Autodesk Inventor part; units mm, degrees
ref_plane "YZ Plane" through (0, 0, 0) normal (1, 0, 0) x (0, 1, 0)
ref_plane "XZ Plane" through (0, 0, 0) normal (0, 1, 0) x (-1, 0, 0)
ref_plane "XY Plane" through (0, 0, 0) normal (0, 0, 1) x (1, 0, 0)
sketch "Esboço2" plane through (0, 0, 0) normal (0, 0, 1) x (1, 0, 0)
  line L0 (0, 0) -> (57, 0)
  line L1 (57, 0) -> (57, 125)
  line L2 (74, 135) -> (74, 161)
  line L3 (74, 161) -> (73, 161)
  line L4 (57, 125) -> (74, 135)
  line L5 (73, 135.5719) -> (56, 125.5719)
  line L6 (56, 125.5719) -> (56, 1)
  line L7 (56, 1) -> (1, 1)
  line L8 (1, 1) -> (0, 1)
  line L9 (0, 1) -> (0, 0)
  line L10 (0, 45.3298) -> (0, 108.1085)
  line L11 (73, 160) -> (73, 161)
  line L12 (73, 138.8946) -> (0.9659, 119.5931)
  line L13 (73, 138.8946) -> (148.5752, 138.8946) construction
  line L14 (0.9659, 118.5931) -> (73, 137.8946)
  line L15 (73, 160) -> (73, 138.8946)
  line L16 (73, 137.8946) -> (73, 135.5719)
  line L17 (0.9659, 119.5931) -> (0.9659, 118.5931)
  dimension "d0" = 57
  dimension "d1" = 125
  dimension "d5" = 26
  dimension "d8" = 1
  dimension "d9" = 165
revolve "Revolução1" add sketch "Esboço2" angle 360 about axis through (0, 45.3298, 0) along (0, 1, 0)
sketch "Esboço3" plane through (0, 0, 0) normal (0, -1, 0) x (1, 0, 0)
  circle A0 centre (0, 0) radius 2.5
  dimension "d13" = 5
extrude "Extrusão1" cut sketch "Esboço3" against normal blind 10
sketch "Esboço4" plane through (0, 0, 0) normal (0, -1, 0) x (1, 0, 0)
  circle A0 centre (0, 0) radius 57
  line L0 (107, 0) -> (107, 32.5)
  line L1 (107, 32.5) -> (107, -32.5)
  line L2 (107, -32.5) -> (27, -32.5)
  line L3 (27, -32.5) -> (107, -32.5)
  line L4 (107, -32.5) -> (107, 32.5)
  line L5 (107, 32.5) -> (27, 32.5)
  line L6 (27, 32.5) -> (27, -32.5)
  point P0 (0, 0)
  dimension "d17" = 32.5
  dimension "d18" = 65
  dimension "d19" = 80
extrude "Extrusão2" add sketch "Esboço4" along normal blind 2 contours A0 L2 L6 L5 | A0 L5 L0 L1 L2 picked at (37, 0)
sketch "Esboço5" plane through (27, 0, 32.5) normal (0, -1, 0) x (1, 0, 0)
  circle A0 centre (-27, -32.5) radius 2.5
  line L0 (-27, -32.5) -> (-65, -32.5)
  circle A1 centre (-65, -32.5) radius 2.5
  dimension "d22" = 38
  dimension "d23" = 5
extrude "Extrusão3" cut sketch "Esboço5" along normal mid plane 6 contours A1
pattern_circular "Padrão circular1" count 4 over 360 about axis through (0, 0, 0) along (0, 1, 0) of "Extrusão3"
sketch "Esboço6" plane through (0, -2, 0) normal (0, -1, 0) x (1, 0, 0)
  line L0 (107, -32.5) -> (107, 32.5)
  line L1 (107, 0) -> (90, 0)
  line L2 (90, 0) -> (90, 20)
  line L3 (90, 0) -> (90, -20)
  circle A0 centre (90, -20) radius 3.5
  circle A1 centre (90, 20) radius 3.5
  point P0 (0, 0)
  dimension "d29" = 17
  dimension "d30" = 20
  dimension "d31" = 20
  dimension "d32" = 7
  dimension "d33" = 7
extrude "Extrusão4" cut sketch "Esboço6" against normal blind 6
sketch "Esboço7" plane through (0, 0, 0) normal (0, 1, 0) x (1, 0, 0)
  arc A0 (46.8268, -32.5) -> (46.8268, 32.5) centre (0, 0) ccw
  line L0 (57, 0) -> (57, -32.5)
  line L1 (46.8268, -32.5) -> (107, -32.5)
  line L2 (57, 0) -> (89.5, 0) construction
  line L3 (57, -32.5) -> (57, -27.5)
  line L4 (57, -27.5) -> (77, -27.5)
  line L5 (77, -27.5) -> (77, -17.5)
  line L6 (77, -17.5) -> (67, -17.5)
  circle A1 centre (67, -17.5) radius 10
  point P0 (0, 0)
  dimension "d36" = 90
  dimension "d37" = 5
  dimension "d38" = 20
  dimension "d39" = 10
  dimension "d40" = 10
extrude "Extrusão5" add sketch "Esboço7" along normal blind 6 contours A1
properties part number "pluviometro"
Could you check a few things on this model? Use its own coordinates, in mm. A direction names the side the tool comes from. Round coordinates to 2 decimals unless told otherwise and drop trailing zeros. Loops run counter-clockwise (first coordinate to the right, second up) from the corner with the lowest first, then second, coordinate; pieces in that order, holes last. Notation, with made-up numbers: (-26, 58.25) - (3, 58.25) arc R12 cw to (3, 73.25) - close; hole circle Ø6 at (-5.5, 81.5). An arc over 180 degrees is marked (long way). Answer in a Markdown table with one row per item. Add a question column.
(1) I need wall thicknesses on line 1 along Z through (x, y) = (90, -1); line 2 along X through (y, z) = (-1, 20); line 3 along Y through (x, z) = (61, 14). Which ranges of each line are inside material? Lowest first, please.
(2) If we section it at C-C (y = 34): Please give me the cut outline in (x, z).
(3) For faces 1 (the face through (-15.825, 149.793, -71.264)), 2 (the face through (51.73, 62.41, -21.45)), 3 (the face through (-0.54, 0.49, -2.44)), which set-ups out of +Z, -Z, +X, -X, +Y, -Y let a thin tool reach every point of the face, with its end or its side?
(4) If we section it at B-B (z = -20): State how many separate pieces and enclosed holes the cut face has, plus the area to 3 significant figures.
(5) I'm going to push flat-ended pins straight in: pin 1 (1.5 mm diameter, centred on x = -48.5, y = 100, fed in from -Z); pin 2 (2 mm diameter, centred on y = -1.5, z = -6.5, fed in from -X); pin 3 (6 mm diameter, centred on x = 38, z = 0, fed in from +Y); pin 4 (10 mm diameter, centred on x = 67.5, z = 17, fed in from +Y). Where does each tip first touch, or does it pass through?
(6) If we mould it in two halves opening along Z, with no side actions, what happens to faces 4 (the face through (35.69, -0.52, 0.96)), 5 (the face through (83, 0, 0)), 6 (the face through (-1.19, 120.8, 5.34)), 7 (the face through (52.654, 63.375, 21.831))? For each: pulls with the +Z half, pulls with the -Z half, needs draft (parallel to the pull), parting line crosses it, or undercut.
(7) If we section it at A-A (x = 90): Please give me the cut outline in (y, z).
Model answer:
| question | item | result |
|---|---|---|
| 1 | line 1 | z = -32.5 to -23.5, -16.5 to 16.5, 23.5 to 32.5 |
| 1 | line 2 | x = 27 to 86.5, 93.5 to 107 |
| 1 | line 3 | y = -2 to 6, 128.29 to 129.45, 135.1 to 136.1 |
| 2 | outline | circle Ø114 at (0, 0); hole circle Ø112 at (0, 0) |
| 3 | face 1 | +Y |
| 3 | face 2 | none |
| 3 | face 3 | -Y |
| 4 | separate pieces | 2 |
| 4 | enclosed holes | 1 |
| 4 | area | 754 mm² |
| 5 | pin 1 | stops at z = -31.13 |
| 5 | pin 2 | stops at x = 27 |
| 5 | pin 3 | stops at y = 130.32 |
| 5 | pin 4 | stops at y = 161 |
| 6 | face 4 | undercut |
| 6 | face 5 | needs draft |
| 6 | face 6 | undercut |
| 6 | face 7 | parting line crosses it |
| 7 | outline | (-2, -32.5) - (0, -32.5) - (0, -23.5) - (-2, -23.5) - close; (-2, -16.5) - (0, -16.5) - (0, 16.5) - (-2, 16.5) - close; (-2, 23.5) - (0, 23.5) - (0, 32.5) - (-2, 32.5) - close |
